Here's the drawing with two shaded views (mm, measured from the low corner). I have some questions. A direction names the side the tool comes from. Coordinates: 2 decimals unless noted, no trailing zeros.
Item 1: If I drill on probe 1 along Y at (x, z) = (8, 7.5) (1 decimal); probe 2 along Y at (x, z) = (9.5, 30) (1 decimal); probe 3 along Z at (x, y) = (14.5, 23.25), over which ranges is the centre line in solid material (lowest first)?
Item 2: Thinking about a two-plate mould opening in Y: for the marked faces 4, 5 and 6, which applies, +Y half, -Y half, draft (parallel to the pull), parting line (faces both ways), or undercut?
Item 3: Which directions (+Z, -Z, +X, -X, +Y, -Y) give clear straight access to the entire face, cutting with the end or side of a thin tool? Please do the marked faces 1, 2 and 3.
Item 4: For P1, Ø3.5, axis at y = 2, z = 6.5, coming from the +X side; P2, Ø4, axis at x = 36.5, y = 14, coming from the +Z side; P3, Ø10, axis at x = 30.5, y = 12, coming from the -Z side, each with a flat end and sliding along its axis, tell me the tip position at first contact or that it passes through.
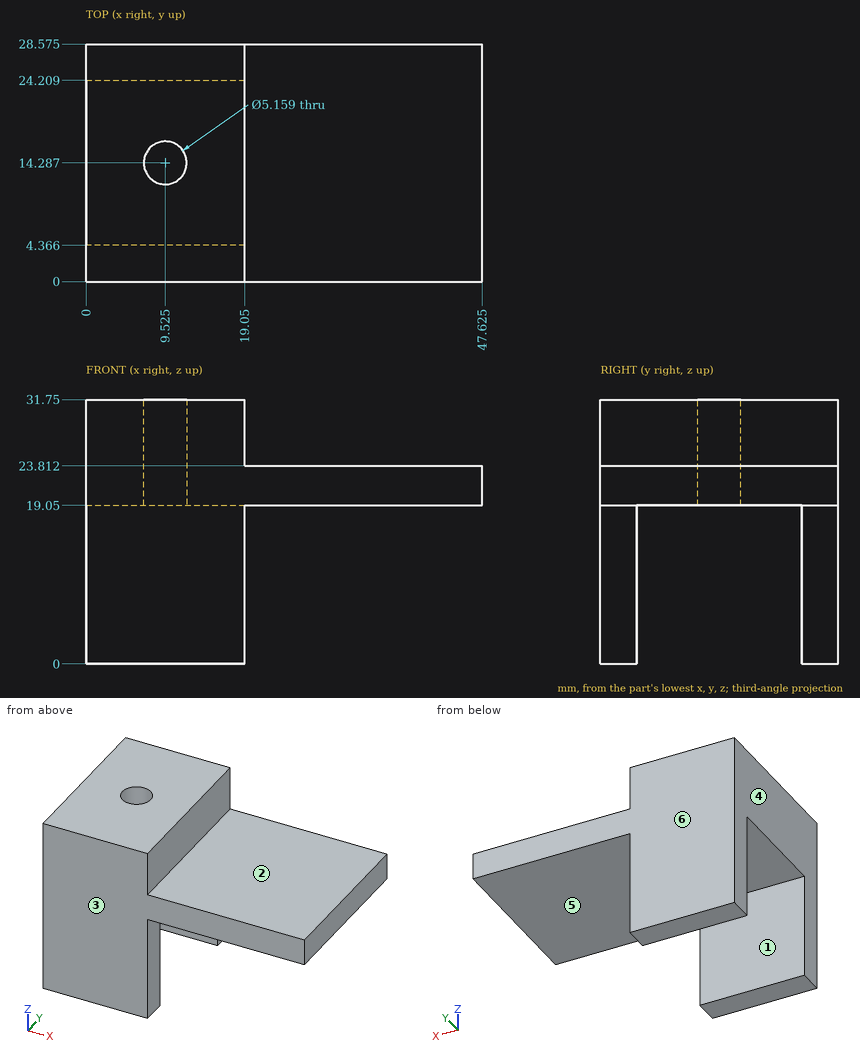
Response values:
1. probe 1: y = 0 to 4.4, 24.2 to 28.6
1. probe 2: y = 0 to 11.7, 16.9 to 28.6
1. probe 3: z = 19.05 to 31.75
2. face 4: draft
2. face 5: undercut
2. face 6: +Y half
3. face 1: -Z, +X, -X
3. face 2: +Z, +X, +Y, -Y
3. face 3: +Z, -Z, +X, -X, -Y
4. P1: stops at x = 19.05
4. P2: stops at z = 23.81
4. P3: stops at z = 19.05
